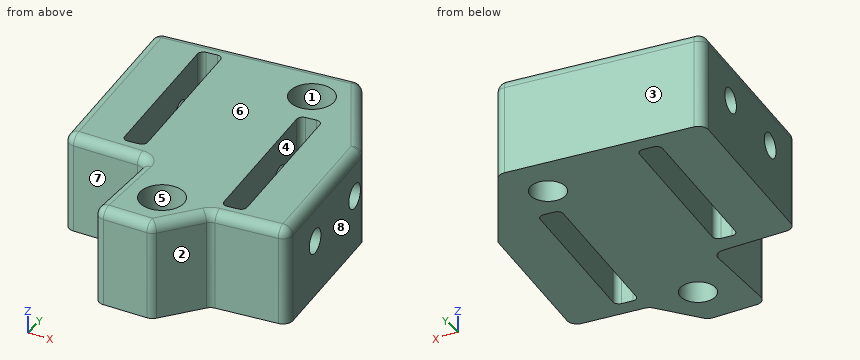
```python
from build123d import *

# Parameters (mm, degrees)
BOSS_EXTRUDE1_DEPTH                      = 12.7
FILLET1_R                                = 1.27
CUT_EXTRUDE1_DEPTH                       = 13.7
FILLET2_R                                = 0.762
F_1_8_0_1250_DOWEL_HOLE1_D               = 3.175
F_1_8_0_1250_DOWEL_HOLE1_DEPTH           = 15.875
F_1_8_0_1250_DOWEL_HOLE1_TIP             = 0.953866233
F_1_8_0_1250_DOWEL_HOLE1_ON_FACE_2_D     = 3.175
F_1_8_0_1250_DOWEL_HOLE1_ON_FACE_2_DEPTH = 15.875
F_1_8_0_1250_DOWEL_HOLE1_ON_FACE_2_TIP   = 0.953866233
F_1_8_0_1250_DOWEL_HOLE1_ON_FACE_3_D     = 3.175
F_1_8_0_1250_DOWEL_HOLE1_ON_FACE_3_DEPTH = 15.875
F_1_8_0_1250_DOWEL_HOLE1_ON_FACE_3_TIP   = 0.953866233
F_1_8_0_1250_DOWEL_HOLE1_ON_FACE_4_D     = 3.175
F_1_8_0_1250_DOWEL_HOLE1_ON_FACE_4_DEPTH = 15.875
F_1_8_0_1250_DOWEL_HOLE1_ON_FACE_4_TIP   = 0.953866233
F_8_CLEARANCE_HOLE1_D                    = 4.4958
F_8_CLEARANCE_HOLE1_DEPTH                = 16.002
F_8_CLEARANCE_HOLE1_TIP                  = 1.350674586
F_2_0_221_DIAMETER_HOLE1_D               = 5.6134
F_2_0_221_DIAMETER_HOLE1_DEPTH           = 4.699
F_2_0_221_DIAMETER_HOLE1_TIP             = 1.686435499


with BuildPart() as part:
    # Sketch1 → Boss-Extrude1 (new body)
    with BuildSketch(Plane.XY):
        Polygon((19.247501297, -20.554356895), (17.457749907, -0.510490359), (10.059696167, 12.303314596), (-15.751947283, 9.998548464), (-13.531962325, -14.863609733), (-2.667, -14.863609733), (-2.667, -27.080616861), (4.953, -27.080616861), (9.525, -21.422495793), align=None)
    extrude(amount=BOSS_EXTRUDE1_DEPTH)

    # Fillet1
    fillet1_edges = [part.edges().sort_by_distance(p)[0] for p in [
        (1.143, -27.080616861, 12.7),
        (-2.667, -20.972113297, 12.7),
        (19.247501297, -20.554356895, 6.35),
        (17.457749907, -0.510490359, 6.35),
        (10.059696167, 12.303314596, 6.35),
        (-15.751947283, 9.998548464, 6.35),
        (-13.531962325, -14.863609733, 6.35),
        (-2.667, -14.863609733, 6.35),
        (-2.667, -27.080616861, 6.35),
        (4.953, -27.080616861, 6.35),
        (9.525, -21.422495793, 6.35),
        (-8.099481163, -14.863609733, 12.7),
        (-14.641954804, -2.432530634, 12.7),
        (-2.846125558, 11.15093153, 12.7),
        (13.758723037, 5.896412118, 12.7),
        (18.352625602, -10.532423627, 12.7),
        (14.386250649, -20.988426344, 12.7),
        (7.239, -24.251556327, 12.7),
    ]]
    fillet(fillet1_edges, radius=FILLET1_R)

    # Sketch2 → Cut-Extrude1 (cut, through all)
    with BuildSketch(Plane.XY.offset(12.7)):
        Polygon((-9.119892735, 8.550651548), (-6.210468147, 8.810439084), (-4.312889622, -12.441010084), (-7.22231421, -12.70079762), align=None)
        Polygon((7.808443636, 1.885201654), (10.717868225, 2.14498919), (12.61544675, -19.106459978), (9.706022161, -19.366247515), align=None)
    extrude(amount=-CUT_EXTRUDE1_DEPTH, mode=Mode.SUBTRACT)

    # Fillet2
    fillet2_edges = [part.edges().sort_by_distance(p)[0] for p in [
        (9.706022161, -19.366247515, 6.35),
        (7.808443636, 1.885201654, 6.35),
        (10.717868225, 2.14498919, 6.35),
        (12.61544675, -19.106459978, 6.35),
        (-7.22231421, -12.70079762, 6.35),
        (-9.119892735, 8.550651548, 6.35),
        (-6.210468147, 8.810439084, 6.35),
        (-4.312889622, -12.441010084, 6.35),
    ]]
    fillet(fillet2_edges, radius=FILLET2_R)

    # 1/8 (0.1250) Dowel Hole1
    with Locations(Plane(origin=(17.637948084, -2.528574118, 7.3025), x_dir=(-0.088937876, 0.996037175, 0), z_dir=(0.996037175, 0.088937876, 0))):
        with Locations((0, 0)):
            Hole(F_1_8_0_1250_DOWEL_HOLE1_D / 2, depth=F_1_8_0_1250_DOWEL_HOLE1_DEPTH)
            with Locations((0, 0, -(F_1_8_0_1250_DOWEL_HOLE1_DEPTH + F_1_8_0_1250_DOWEL_HOLE1_TIP / 2))):  # 118° drill point
                Cone(0, F_1_8_0_1250_DOWEL_HOLE1_D / 2, F_1_8_0_1250_DOWEL_HOLE1_TIP, mode=Mode.SUBTRACT)

    # 1/8 (0.1250) Dowel Hole1 on face 2
    with Locations(Plane(origin=(18.598032457, -13.280795423, 7.3025), x_dir=(-0.088938015, 0.996037163, 0), z_dir=(0.996037163, 0.088938015, 0))):
        with Locations((0, 0)):
            Hole(F_1_8_0_1250_DOWEL_HOLE1_ON_FACE_2_D / 2, depth=F_1_8_0_1250_DOWEL_HOLE1_ON_FACE_2_DEPTH)
            with Locations((0, 0, -(F_1_8_0_1250_DOWEL_HOLE1_ON_FACE_2_DEPTH + F_1_8_0_1250_DOWEL_HOLE1_ON_FACE_2_TIP / 2))):  # 118° drill point
                Cone(0, F_1_8_0_1250_DOWEL_HOLE1_ON_FACE_2_D / 2, F_1_8_0_1250_DOWEL_HOLE1_ON_FACE_2_TIP, mode=Mode.SUBTRACT)

    # 1/8 (0.1250) Dowel Hole1 on face 3
    with Locations(Plane(origin=(-15.102478442, 2.724986993, 7.3025), x_dir=(0.088938015, -0.996037163, 0), z_dir=(-0.996037163, -0.088938015, 0))):
        with Locations((0, 0)):
            Hole(F_1_8_0_1250_DOWEL_HOLE1_ON_FACE_3_D / 2, depth=F_1_8_0_1250_DOWEL_HOLE1_ON_FACE_3_DEPTH)
            with Locations((0, 0, -(F_1_8_0_1250_DOWEL_HOLE1_ON_FACE_3_DEPTH + F_1_8_0_1250_DOWEL_HOLE1_ON_FACE_3_TIP / 2))):  # 118° drill point
                Cone(0, F_1_8_0_1250_DOWEL_HOLE1_ON_FACE_3_D / 2, F_1_8_0_1250_DOWEL_HOLE1_ON_FACE_3_TIP, mode=Mode.SUBTRACT)

    # 1/8 (0.1250) Dowel Hole1 on face 4
    with Locations(Plane(origin=(-14.14239407, -8.027234313, 7.3025), x_dir=(0.088938015, -0.996037163, 0), z_dir=(-0.996037163, -0.088938015, 0))):
        with Locations((0, 0)):
            Hole(F_1_8_0_1250_DOWEL_HOLE1_ON_FACE_4_D / 2, depth=F_1_8_0_1250_DOWEL_HOLE1_ON_FACE_4_DEPTH)
            with Locations((0, 0, -(F_1_8_0_1250_DOWEL_HOLE1_ON_FACE_4_DEPTH + F_1_8_0_1250_DOWEL_HOLE1_ON_FACE_4_TIP / 2))):  # 118° drill point
                Cone(0, F_1_8_0_1250_DOWEL_HOLE1_ON_FACE_4_D / 2, F_1_8_0_1250_DOWEL_HOLE1_ON_FACE_4_TIP, mode=Mode.SUBTRACT)

    # #8 Clearance Hole1
    with Locations(Plane.XY.offset(12.7)):
        with Locations((6.934384891, 6.286512516), (3.048, -21.365616861)):
            Hole(F_8_CLEARANCE_HOLE1_D / 2, depth=F_8_CLEARANCE_HOLE1_DEPTH)
            with Locations((0, 0, -(F_8_CLEARANCE_HOLE1_DEPTH + F_8_CLEARANCE_HOLE1_TIP / 2))):  # 118° drill point
                Cone(0, F_8_CLEARANCE_HOLE1_D / 2, F_8_CLEARANCE_HOLE1_TIP, mode=Mode.SUBTRACT)

    # #2 (0.221) Diameter Hole1
    with Locations(Plane.XY.offset(12.7)):
        with Locations((6.934384891, 6.286512516), (3.048, -21.365616861)):
            Hole(F_2_0_221_DIAMETER_HOLE1_D / 2, depth=F_2_0_221_DIAMETER_HOLE1_DEPTH)
            with Locations((0, 0, -(F_2_0_221_DIAMETER_HOLE1_DEPTH + F_2_0_221_DIAMETER_HOLE1_TIP / 2))):  # 118° drill point
                Cone(0, F_2_0_221_DIAMETER_HOLE1_D / 2, F_2_0_221_DIAMETER_HOLE1_TIP, mode=Mode.SUBTRACT)


solid = part.part
```
Verification items for the finished model (mm, model axes). Face numbers are marked on the shaded views. A direction names the side the tool comes from. Round coordinates to 2 decimals unless told otherwise and drop trailing zeros.
1. Gauge pin test, flat ends, axial feed: P1, Ø5, axis at y = -4, z = 9.5, coming from the +X side; P2, Ø2, axis at y = -13, z = 8, coming from the -X side; P3, Ø3, axis at y = -11.5, z = 4.5, coming from the -X side. Record the tip position at first contact, or that the pin passes through.
2. Draft check along Y on the marked faces 1, 2 and 3. Enter one of: +Y half, -Y half, draft (parallel to the pull), parting line (faces both ways), or undercut.
3. Access from +Z, -Z, +X, -X, +Y, -Y to the whole of each face (thin tool, end or side, straight path). Record for the marked faces 4, 5, 6, 7 and 8.
4. Scan lines: L1, parallel to X at y = -5, z = 10.25; L2, parallel to Y at x = 3, z = 6.5; L3, parallel to X at y = 6, z = 10. Record each from-to range of solid material in increasing order.
5. Section check A-A on z = 6.75. State how many separate pieces and enclosed holes the cut face has, plus the area to 3 significant figures.
Answer:
1. P1: stops at x = 17.99
1. P2: stops at x = -13.79
1. P3: stops at x = -13.97
2. face 1: undercut
2. face 2: -Y half
2. face 3: +Y half
3. face 4: +Z, -Z
3. face 5: +Z
3. face 6: +Z, +X, -X, +Y, -Y
3. face 7: +Z, -Z, -X, -Y
3. face 8: +Z, -Z, +X, +Y
4. L1: x = -14.41 to -7.91, -4.98 to 8.42, 11.36 to 17.86
4. L2: y = -27.08 to -23.61, -19.12 to -16.05, -13.3 to -5.21, -2.46 to 11.67
4. L3: x = -15.39 to -8.89, -5.96 to 4.14, 9.73 to 13.7
5. separate pieces: 3
5. enclosed holes: 2
5. area: 686 mm2
